from build123d import *

# Parameters (mm, degrees)
SKETCH1_R                 = 12.2
BOSS_EXTRUDE1_DEPTH       = 47
BOSS_EXTRUDE2_START       = 47
SKETCH1_3_R               = 12.5
SKETCH1_3_R_2             = 12.2
BOSS_EXTRUDE2_DEPTH       = 19
SKETCH2_R                 = 3.5
SKETCH2_R_2               = 2
BOSS_EXTRUDE4_DEPTH       = 2.5
BOSS_EXTRUDE5_START       = 2.5
BOSS_EXTRUDE5_DEPTH       = 11
M3X0_5_TAPPED_HOLE1_D     = 2.5
M3X0_5_TAPPED_HOLE1_DEPTH = 20
M3X0_5_TAPPED_HOLE1_TIP   = 0.751075774


with BuildPart() as part:
    # Sketch1 → Boss-Extrude1 (new body)
    with BuildSketch(Plane.XY):
        Circle(SKETCH1_R)
    extrude(amount=BOSS_EXTRUDE1_DEPTH)

    # Sketch1<3> → Boss-Extrude2 (add)
    with BuildSketch(Plane.XY.offset(BOSS_EXTRUDE2_START)):
        Circle(SKETCH1_3_R)
        Circle(SKETCH1_3_R_2, mode=Mode.SUBTRACT)
        Circle(SKETCH1_3_R_2)
    extrude(amount=BOSS_EXTRUDE2_DEPTH)

    # Sketch2 → Boss-Extrude4 (add)
    with BuildSketch(Plane.XY.offset(66)):
        Circle(SKETCH2_R)
        Circle(SKETCH2_R_2, mode=Mode.SUBTRACT)
        with BuildLine():
            Line((1.322875656, 1.5), (-1.322875656, 1.5))
            ThreePointArc((-1.322875656, 1.5), (-0.822875656, -1.822875656), (2, 0))
            ThreePointArc((2, 0), (1.822875656, 0.822875656), (1.322875656, 1.5))
        make_face()
        with BuildLine():
            ThreePointArc((1.322875656, 1.5), (0, 2), (-1.322875656, 1.5))
            Line((-1.322875656, 1.5), (1.322875656, 1.5))
        make_face()
    extrude(amount=BOSS_EXTRUDE4_DEPTH)

    # Sketch2<4> → Boss-Extrude5 (add)
    with BuildSketch(Plane.XY.offset(66).offset(BOSS_EXTRUDE5_START)):
        with BuildLine():
            Line((1.322875656, 1.5), (-1.322875656, 1.5))
            ThreePointArc((-1.322875656, 1.5), (-0.822875656, -1.822875656), (2, 0))
            ThreePointArc((2, 0), (1.822875656, 0.822875656), (1.322875656, 1.5))
        make_face()
    extrude(amount=BOSS_EXTRUDE5_DEPTH)

    # M3x0.5 Tapped Hole1
    with Locations(Plane(origin=(0, 8.75, 66), x_dir=(1, 0, 0), z_dir=(0, 0, 1))):
        with Locations((0, 0), (0, -17.5)):
            Hole(M3X0_5_TAPPED_HOLE1_D / 2, depth=M3X0_5_TAPPED_HOLE1_DEPTH)
            with Locations((0, 0, -(M3X0_5_TAPPED_HOLE1_DEPTH + M3X0_5_TAPPED_HOLE1_TIP / 2))):  # 118° drill point
                Cone(0, M3X0_5_TAPPED_HOLE1_D / 2, M3X0_5_TAPPED_HOLE1_TIP, mode=Mode.SUBTRACT)


solid = part.part
The model under review builds one solid part; all positions refer to its coordinate system, in mm. A direction names the side the tool comes from. Coordinates: 2 decimals unless noted, no trailing zeros. Write each loop counter-clockwise with the first axis right and the second up, starting at its lowest first coordinate (ties: lowest second). Pieces come first, ordered by that corner, then holes. Notation, with made-up numbers: (8, 52.25) - (62, 52.25) arc R23 cw to (62, 83.25) - close; hole circle Ø5 at (-26, 36). An arc over 180 degrees is marked (long way). Answer as a JSON object with one key per item and string values. Group by question number.
1. Add section D-D (z = 38). Give the boundary of the cut face in (x, y).
2. Add section A-A (y = -11). Give the boundary of the cut face in (x, z).
3. Mouldability with a two-part tool opening along X and no side actions: class faces 1 (the face through (0.2, -8.83, 45.38)), 2 (the face through (3.233, -1.341, 67.232)), 3 (the face through (3, -3, 66)) as pulls with the +X half, pulls with the -X half, needs draft (parallel to the pull), parting line crosses it, or undercut.
4. To check wall thickness, follow probe 1 along Y at (x, z) = (0, 61.25); probe 2 along Z at (x, y) = (3.5, 8.5); probe 3 along X at (y, z) = (-8.5, 61). State the ranges of each line that lie inside material, in increasing order.
5. Machinability: for faces 4 (the face through (0, 1.5, 74)), 5 (the face through (0, 0, 0)), 6 (the face through (0, 0, 79.5)), 7 (the face through (-0.672, 9.804, 55.86)), 8 (the face through (-12.19, 0.54, 23.17)), which of the approach directions +Z, -Z, +X, -X, +Y, -Y give a long, thin tool a straight path to every point of the face, cutting with its end or side? Answer none if there is none.
6. Clearance check with flat-ended pins moving along their axes: pin 1 Ø2 at (x, z) = (0, 75.5) entering from +Y; pin 2 Ø5 at (x, y) = (-8.5, -7) entering from +Z; pin 3 Ø6 at (x, z) = (-1, 20.5) entering from -Y; pin 4 Ø1.5 at (y, z) = (8.5, 67) entering from +X. State where each tip first meets the part, or that it passes through.
7. Add section B-B (z = 71). Give the boundary of the cut face in (x, y), plus the area to 3 significant figures.
8. Add section C-C (x = 5.25). Give the boundary of the cut face in (y, z), plus the area to 3 significant figures.
Findings:
{
 "1": {"outline": "circle Ø24.4 at (0, 0)"},
 "2": {"outline": "(-5.94, 47) - (-5.28, 47) - (-5.28, 0) - (5.28, 0) - (5.28, 47) - (5.94, 47) - (5.94, 66) - (-5.94, 66) - close"},
 "3": {"face 1": "undercut", "face 2": "parting line crosses it", "face 3": "needs draft"},
 "4": {"probe 1": "-12.5 to -10, -7.5 to 7.5, 10 to 12.5", "probe 2": "0 to 66", "probe 3": "-9.17 to -1.22, 1.22 to 9.17"},
 "5": {"face 4": "+Z, +X, -X, +Y", "face 5": "-Z, +X, -X, +Y, -Y", "face 6": "+Z, +X, -X, +Y, -Y", "face 7": "+Z", "face 8": "-Z"},
 "6": {"pin 1": "y = 1.5", "pin 2": "z = 66", "pin 3": "y = -12.2", "pin 4": "through"},
 "7": {"outline": "(-1.32, 1.5) arc R2 ccw (long way) to (1.32, 1.5) - close", "area": "11.7 mm²"},
 "8": {"outline": "(-11.34, 47) - (-11.01, 47) - (-11.01, 0) - (11.01, 0) - (11.01, 47) - (11.34, 47) - (11.34, 66) - (-11.34, 66) - close", "area": "1,470 mm²"}
}
